```python
from build123d import *

# Parameters (mm, degrees)
SKETCH_1_W             = 30
SKETCH_1_H             = 30
EXTRUDE_398_DEPTH      = 5.35
SKETCH_2_R             = 1.75
CUT_EXTRUDE_618_DEPTH  = 24.758998295
SKETCH_4_W             = 15
SKETCH_4_H             = 15
CUT_EXTRUDE_1118_DEPTH = 24.758998295
FILLET_3_R             = 5
FILLET_6_R             = 4


with BuildPart() as part:
    # Эскиз1 → Extrude 398 (new, symmetric)
    with BuildSketch(Plane(origin=(0, 0, 0), x_dir=(1, 0, 0), z_dir=(0, 1, 0))):
        Rectangle(SKETCH_1_W, SKETCH_1_H)
    extrude(amount=EXTRUDE_398_DEPTH, both=True)

    # Эскиз2 → Cut-Extrude 618 (cut, through all)
    with BuildSketch(Plane(origin=(0, -5.35, 0), x_dir=(1, 0, 0), z_dir=(0, 1, 0))):
        with Locations(Location((-10, 10, 0), (0, 0, 270))):
            Circle(SKETCH_2_R)
        with Locations(Location((10, 10, 0), (0, 0, 270))):
            Circle(SKETCH_2_R)
        with Locations(Location((10, -10, 0), (0, 0, 270))):
            Circle(SKETCH_2_R)
        with Locations(Location((-10, -10, 0), (0, 0, 270))):
            Circle(SKETCH_2_R)
    extrude(amount=CUT_EXTRUDE_618_DEPTH, mode=Mode.SUBTRACT)

    # Эскиз4 → Cut-Extrude 1118 (cut, through all)
    with BuildSketch(Plane(origin=(0, 5.35, 0), x_dir=(1, 0, 0), z_dir=(0, 1, 0))):
        Rectangle(SKETCH_4_W, SKETCH_4_H)
    extrude(amount=-CUT_EXTRUDE_1118_DEPTH, mode=Mode.SUBTRACT)

    # Скругление3
    fillet_3_edges = [part.edges().sort_by_distance(p)[0] for p in [
        (-7.5, 0, 7.5),
        (-7.5, 0, -7.5),
        (7.5, 0, -7.5),
        (7.5, 0, 7.5),
    ]]
    fillet(fillet_3_edges, radius=FILLET_3_R)

    # Скругление6
    fillet_6_edges = [part.edges().sort_by_distance(p)[0] for p in [
        (15, 0, 15),
        (-15, 0, 15),
        (-15, 0, -15),
        (15, 0, -15),
    ]]
    fillet(fillet_6_edges, radius=FILLET_6_R)


solid = part.part
```
Here's how the part is built. I have some questions about the finished solid (model axes, mm). A direction names the side the tool comes from. Give positions to 0.01 mm unless a question says otherwise; leave off trailing zeros. Write each loop counter-clockwise with the first axis right and the second up, starting at its lowest first coordinate (ties: lowest second). Pieces come first, ordered by that corner, then holes.
(1) Thinking about a two-plate mould opening in X: for faces 1 (the face through (0, 0, 7.5)), 2 (the face through (-7, 5.35, -7)), 3 (the face through (-8.5, -0.1, -9.1)), 4 (the face through (-13.859, -0.075, -13.797)), which applies, pulls with the +X half, pulls with the -X half, needs draft (parallel to the pull), parting line crosses it, or undercut?
Output values:
face 1: undercut
face 2: needs draft
face 3: undercut
face 4: pulls with the -X half
(2) If I drill on L1, parallel to Z at x = -10, y = -0.75; L2, parallel to X at y = 0, z = 0, over which ranges is the centre line in solid material (lowest first)?
Output values:
L1: z = -15 to -11.75, -8.25 to 8.25, 11.75 to 15
L2: x = -15 to -7.5, 7.5 to 15
(3) On a 3-axis mill with a long thin cutter (end or side, diameter ignored), from which of +Z, -Z, +X, -X, +Y, -Y can I reach the whole of each face in a straight line? I mean faces 5 (the face through (0, 0, -7.5)), 6 (the face through (-13.859, 0.075, 13.797)). Say none if no direction works.
Output values:
face 5: +Y, -Y
face 6: +Z, -X, +Y, -Y
(4) Will this pin go through, and if not, where does the flat tip stop? pin 1 (3 mm diameter, centred on x = 2.5, z = 4, fed in from +Y).
Output values:
pin 1: passes through
(5) Imagine slicing it at C-C, the plane y = -1. Write out the boundary of the cut face in (x, z), and give its area (3 significant figures).
Output values:
outline: (-15, -11) arc R4 ccw to (-11, -15) - (11, -15) arc R4 ccw to (15, -11) - (15, 11) arc R4 ccw to (11, 15) - (-11, 15) arc R4 ccw to (-15, 11) - close; hole circle Ø3.5 at (-10, -10); hole circle Ø3.5 at (-10, 10); hole (-7.5, -2.5) arc R5 ccw to (-2.5, -7.5) - (2.5, -7.5) arc R5 ccw to (7.5, -2.5) - (7.5, 2.5) arc R5 ccw to (2.5, 7.5) - (-2.5, 7.5) arc R5 ccw to (-7.5, 2.5) - close; hole circle Ø3.5 at (10, -10); hole circle Ø3.5 at (10, 10)
area: 644 mm2
(6) Imagine slicing it at B-B, the plane z = 10. Write out the boundary of the cut face in (x, y), and give its area (3 significant figures).
Output values:
outline: (-15, -5.35) - (-11.75, -5.35) - (-11.75, 5.35) - (-15, 5.35) - close; (-8.25, -5.35) - (8.25, -5.35) - (8.25, 5.35) - (-8.25, 5.35) - close; (11.75, -5.35) - (15, -5.35) - (15, 5.35) - (11.75, 5.35) - close
area: 246 mm2
(7) Imagine slicing it at D-D, the plane z = 0. Write out the boundary of the cut face in (x, y), and give its area (4 significant figures).
Output values:
outline: (-15, -5.35) - (-7.5, -5.35) - (-7.5, 5.35) - (-15, 5.35) - close; (7.5, -5.35) - (15, -5.35) - (15, 5.35) - (7.5, 5.35) - close
area: 160.5 mm2
(8) Imagine slicing it at A-A, the plane x = -10. Write out the boundary of the cut face in (y, z), and give its area (3 significant figures).
Output values:
outline: (-5.35, -15) - (5.35, -15) - (5.35, -11.75) - (-5.35, -11.75) - close; (-5.35, -8.25) - (5.35, -8.25) - (5.35, 8.25) - (-5.35, 8.25) - close; (-5.35, 11.75) - (5.35, 11.75) - (5.35, 15) - (-5.35, 15) - close
area: 246 mm2
